Geometry: final body of the model. Coordinates: model frame, mm. Give positions to 0.01 mm unless a question says otherwise; leave off trailing zeros. Write each loop counter-clockwise with the first axis right and the second up, starting at its lowest first coordinate (ties: lowest second). Pieces come first, ordered by that corner, then holes. Notation, with made-up numbers: M 26,-33.75 L 46,-33.75 A37 ccw 46,2.25 Z; hole C -24,-10.75 d8. An arc over 180 degrees is marked long. Answer as a JSON object with one key per item and string values.
from build123d import *

# Parameters (mm, degrees)
SKETCH1_W           = 77
SKETCH1_H           = 26
BOSS_EXTRUDE1_DEPTH = 2
SKETCH2_R           = 1.5
CUT_EXTRUDE1_DEPTH  = 2
SKETCH3_R           = 0.51
CUT_EXTRUDE2_DEPTH  = 2


with BuildPart() as part:
    # Sketch1 → Boss-Extrude1 (new body)
    with BuildSketch(Plane(origin=(0, 0, 0), x_dir=(1, 0, 0), z_dir=(0, 1, 0))):
        with Locations((38.5, -13)):
            Rectangle(SKETCH1_W, SKETCH1_H)
    extrude(amount=BOSS_EXTRUDE1_DEPTH)

    # Sketch2 → Cut-Extrude1 (cut)
    with BuildSketch(Plane(origin=(0, 2, 0), x_dir=(1, 0, 0), z_dir=(0, 1, 0))):
        with Locations(Location((3.5, -22.5, 0), (0, 0, 270))):
            Circle(SKETCH2_R)
        with Locations(Location((73.5, -22.5, 0), (0, 0, 270))):
            Circle(SKETCH2_R)
    extrude(amount=-CUT_EXTRUDE1_DEPTH, mode=Mode.SUBTRACT)

    # Sketch3 → Cut-Extrude2 (cut)
    with BuildSketch(Plane(origin=(0, 2, 0), x_dir=(1, 0, 0), z_dir=(0, 1, 0))):
        with Locations(Location((27.07, -24.179660029, 0), (0, 0, 270))):
            Circle(SKETCH3_R)
        with Locations(Location((29.61, -24.179660029, 0), (0, 0, 270))):
            Circle(SKETCH3_R)
        with Locations(Location((32.15, -24.179660029, 0), (0, 0, 270))):
            Circle(SKETCH3_R)
        with Locations(Location((34.69, -24.179660029, 0), (0, 0, 270))):
            Circle(SKETCH3_R)
        with Locations(Location((37.23, -24.179660029, 0), (0, 0, 270))):
            Circle(SKETCH3_R)
        with Locations(Location((39.77, -24.179660029, 0), (0, 0, 270))):
            Circle(SKETCH3_R)
        with Locations(Location((42.31, -24.179660029, 0), (0, 0, 270))):
            Circle(SKETCH3_R)
        with Locations(Location((44.85, -24.179660029, 0), (0, 0, 270))):
            Circle(SKETCH3_R)
        with Locations(Location((47.39, -24.179660029, 0), (0, 0, 270))):
            Circle(SKETCH3_R)
        with Locations(Location((49.93, -24.179660029, 0), (0, 0, 270))):
            Circle(SKETCH3_R)
    extrude(amount=-CUT_EXTRUDE2_DEPTH, mode=Mode.SUBTRACT)


solid = part.part
1) Line query: line 1 (Z direction, x = 34.69, y = 0.8); line 2 (Z direction, x = 73.5, y = 1.5). Output: solid intervals per line, ascending. Write a range as from..to.
Geometry check:
{"line 1": "z = 0..23.67, 24.69..26", "line 2": "z = 0..21, 24..26"}
2) Cut plane B-B on z = 22.5. Return loops of the section in (x, y).
Geometry check:
{"outline": "M 0,0 L 2,0 L 2,2 L 0,2 Z; M 5,0 L 72,0 L 72,2 L 5,2 Z; M 75,0 L 77,0 L 77,2 L 75,2 Z"}
3) Pull-direction query (X, two-part tool) for faces 1 (the cylindrical face through (3.57, 1.01, 21)), 2 (the flat face through (38, 1, 0)), 3 (the flat face through (77, 1, 13)); classes: pulls with the +X half, pulls with the -X half, needs draft (parallel to the pull), parting line crosses it, or undercut.
Geometry check:
{"face 1": "undercut", "face 2": "needs draft", "face 3": "pulls with the +X half"}
4) Contact query for a flat-ended pin moving along its axis: P1, Ø1.6, axis at x = 27.07, z = 24.18, coming from the -Y side. Output: stop coordinate, or through.
Geometry check:
{"P1": "stops at y = 0"}
5) Cut plane A-A on x = 3.5. Return loops of the section in (y, z), and give its area (3 significant figures).
Geometry check:
{"outline": "M 0,0 L 2,0 L 2,21 L 0,21 Z; M 0,24 L 2,24 L 2,26 L 0,26 Z", "area": "46.0 mm2"}
